Part model, mm, in its own coordinate system. Give positions to 0.01 mm unless a question says otherwise; leave off trailing zeros. Return JSON: item names as keys, results as strings.
from build123d import *

# Parameters (mm, degrees)
SKETCH1_W           = 387.35
SKETCH1_H           = 330.2
SKETCH1_R           = 3.96875
BOSS_EXTRUDE1_DEPTH = 3.9878


with BuildPart() as part:
    # Sketch1 → Boss-Extrude1 (new body)
    with BuildSketch(Plane.XY):
        Rectangle(SKETCH1_W, SKETCH1_H)
        with Locations((-180.975, 0)):
            Circle(SKETCH1_R, mode=Mode.SUBTRACT)
        with Locations((0, 152.4)):
            Circle(SKETCH1_R, mode=Mode.SUBTRACT)
        with Locations((152.4, 152.4)):
            Circle(SKETCH1_R, mode=Mode.SUBTRACT)
        with Locations((-152.4, 152.4)):
            Circle(SKETCH1_R, mode=Mode.SUBTRACT)
        with Locations(Location((180.975, 0, 0), (0, 0, 180))):
            Circle(SKETCH1_R, mode=Mode.SUBTRACT)
        with Locations(Location((152.4, -152.4, 0), (0, 0, 180))):
            Circle(SKETCH1_R, mode=Mode.SUBTRACT)
        with Locations(Location((0, -152.4, 0), (0, 0, 180))):
            Circle(SKETCH1_R, mode=Mode.SUBTRACT)
        with Locations(Location((-152.4, -152.4, 0), (0, 0, 180))):
            Circle(SKETCH1_R, mode=Mode.SUBTRACT)
    extrude(amount=BOSS_EXTRUDE1_DEPTH)


solid = part.part
Q1. Probe line 1 along Y through (x, z) = (-152.4, 1.25); line 2 along X through (y, z) = (-152.4, 1.75) (3 decimals). List the from-to ranges inside material, lowest first.
Established:
{"line 1": "y = -165.1 to -156.37, -148.43 to 148.43, 156.37 to 165.1", "line 2": "x = -193.675 to -156.369, -148.431 to -3.969, 3.969 to 148.431, 156.369 to 193.675"}
Q2. Pin check, flat tips, straight feed: pin 1 (2 mm diameter, centred on x = -115, y = 82, fed in from -Z); pin 2 (6.5 mm diameter, centred on x = 180.975, y = 0, fed in from +Z). Stop position of each tip, or through.
Established:
{"pin 1": "stops at z = 0", "pin 2": "passes through"}
Q3. Two-plate mould, pull along X, no slides. Class faces 1 (the flat face through (-3, 2, 0)), 2 (the cylindrical face through (-149.251, -149.985, 1.966)), 3 (the cylindrical face through (148.734, -150.88, 1.966)): +X half, -X half, draft (parallel to the pull), parting line (faces both ways), or undercut.
Established:
{"face 1": "draft", "face 2": "undercut", "face 3": "undercut"}
